```python
from build123d import *

# Parameters (mm, degrees)
SKETCH2_R          = 4.25
CUT_EXTRUDE1_DEPTH = 26.734218465
CHAMFER1_SIZE      = 1
CUT_EXTRUDE2_DEPTH = 26.734218465
CIRPATTERN1_COUNT  = 4


with BuildPart() as part:
    # Sketch1 → Revolve1 (revolve)
    with BuildSketch(Plane.XY, mode=Mode.PRIVATE) as revolve1_sk:
        with BuildLine():
            Line((0, 20.5), (-8, 20.5))
            ThreePointArc((-8, 20.5), (-9.532088886, 19.785575219), (-9.969615506, 18.152703645))
            Line((-9.969615506, 18.152703645), (-8.769638586, 11.347296355))
            ThreePointArc((-8.769638586, 11.347296355), (-9.207165206, 9.714424781), (-10.739254092, 9))
            Line((-10.739254092, 9), (-11, 9))
            Line((-11, 9), (-11, 4))
            Line((-11, 4), (-9.5, 0))
            Line((-9.5, 0), (-8.75, 0))
            Line((-8.75, 0), (0, 8.75))
            Line((0, 8.75), (0, 20.5))
        make_face()
    revolve(revolve1_sk.sketch.rotate(Axis((0, 20.5, 0), (0, -1, 0)), 270), axis=Axis((0, 20.5, 0), (0, -1, 0)))

    # Sketch2 → Cut-Extrude1 (cut, through all)
    with BuildSketch(Plane(origin=(0, 20.5, 0), x_dir=(1, 0, 0), z_dir=(0, 1, 0))):
        with Locations(Location((0, 0, 0), (0, 0, 270))):
            Circle(SKETCH2_R)
    extrude(amount=-CUT_EXTRUDE1_DEPTH, mode=Mode.SUBTRACT)

    # Chamfer1
    chamfer1_edges = [part.edges().sort_by_distance(p)[0] for p in [
        (0, 20.5, -4.25),
    ]]
    chamfer(chamfer1_edges, length=CHAMFER1_SIZE)

    # Sketch3 → Cut-Extrude2 (cut, symmetric)
    with BuildSketch(Plane(origin=(0, 0, 0), x_dir=(0, 0, -1), z_dir=(1, 0, 0))):
        with BuildLine():
            Line((-8.5, 20.5), (-6.974294891, 11.847296355))
            ThreePointArc((-6.974294891, 11.847296355), (-7.411821511, 10.214424781), (-8.943910397, 9.5))
            Line((-8.943910397, 9.5), (-13.5, 9.5))
            Line((-13.5, 9.5), (-13.5, 20.5))
            Line((-13.5, 20.5), (-8.5, 20.5))
        make_face()
    cut_extrude2 = extrude(amount=CUT_EXTRUDE2_DEPTH, both=True, mode=Mode.SUBTRACT)

    # CirPattern1: Cut-Extrude2 ×4 about axis
    cirpattern1_axis = Axis((0, 0, 0), (0, 1, 0))
    for i in range(1, CIRPATTERN1_COUNT):
        add(cut_extrude2.rotate(cirpattern1_axis, i * 360 / CIRPATTERN1_COUNT), mode=Mode.SUBTRACT)


solid = part.part
```
Could you check a few things on this model? Use its own coordinates, in mm. A direction names the side the tool comes from. Round coordinates to 2 decimals unless told otherwise and drop trailing zeros. Loops run counter-clockwise (first coordinate to the right, second up) from the corner with the lowest first, then second, coordinate; pieces in that order, holes last. Notation, with made-up numbers: (15, 17) - (58, 17) arc R14 cw to (58, 29) - close; hole circle Ø4 at (54.5, 48.5). An arc over 180 degrees is marked (long way). Answer in a Markdown table with one row per item. Add a question column.
(1) If we section it at B-B (z = 0): Please give me the cut outline in (x, y), plus the area to 3 significant figures.
(2) I'm going to push flat-ended pins straight in: pin 1 (1.5 mm diameter, centred on y = 13.5, z = 3, fed in from -X); pin 2 (2 mm diameter, centred on x = -2, z = 0, fed in from +Y); pin 3 (1.5 mm diameter, centred on x = -5, y = 17, fed in from +Z); pin 4 (2 mm diameter, centred on x = -3.5, y = 2.5, fed in from +Z). Where does each tip first touch, or does it pass through?
(3) If we section it at C-C (y = 17.25): Please give me the cut outline in (x, z), plus the area to 3 significant figures.
(4) If we section it at D-D (y = 10): Please give me the cut outline in (x, z).
(5) For faces 5 (the face through (7.74, 16.2, -0.08)), 6 (the face through (-0.08, 16.2, -7.74)), 7 (the face through (-6.634, 14.702, -6.604)), 8 (the face through (6.604, 14.702, -6.634)), 9 (the face through (-7.74, 16.2, 0.08)), which set-ups out of +Z, -Z, +X, -X, +Y, -Y let a thin tool reach every point of the face, with its end or its side?
(6) If we section it at A-A (x = 0): Please give me the cut outline in (y, z), plus the area to 3 significant figures.
(7) I need wall thicknesses on line 1 along X through (y, z) = (14, -2.5); line 2 along X through (y, z) = (6.25, 2); line 3 along Z through (x, y) = (-1.75, 16). Which ranges of each line are inside material? Lowest first, please.
(8) If we mould it in two halves opening along Y, with no side actions, what happens to faces 1 (the face through (10.74, 6.46, -2.38)), 2 (the face through (-0.08, 10.23, -7.4)), 3 (the face through (-2.875, 0.194, 9.131)), 4 (the face through (1.7, 20.5, -5.2))? For each: pulls with the +Y half, pulls with the -Y half, needs draft (parallel to the pull), parting line crosses it, or undercut.
Model answer:
| question | item | result |
|---|---|---|
| 1 | outline | (-11, 4) - (-9.5, 0) - (-8.75, 0) - (-4.25, 4.5) - (-4.25, 19.5) - (-5.25, 20.5) - (-8, 20.5) arc R2 ccw to (-8.49, 20.44) - (-6.97, 11.85) arc R2 cw to (-8.94, 9.5) - (-9.42, 9.5) arc R2 cw to (-10.74, 9) - (-11, 9) - close; (4.25, 4.5) - (8.75, 0) - (9.5, 0) - (11, 4) - (11, 9) - (10.74, 9) arc R2 cw to (9.42, 9.5) - (8.94, 9.5) arc R2 cw to (6.97, 11.85) - (8.49, 20.44) arc R2 ccw to (8, 20.5) - (5.25, 20.5) - (4.25, 19.5) - close |
| 1 | area | 175 mm² |
| 2 | pin 1 | stops at x = -7.4 |
| 2 | pin 2 | passes through |
| 2 | pin 3 | stops at z = 8.02 |
| 2 | pin 4 | stops at z = 10.34 |
| 3 | outline | (-7.93, -5.78) arc R9.81 ccw to (-5.78, -7.93) - (5.78, -7.93) arc R9.81 ccw to (7.93, -5.78) - (7.93, 5.78) arc R9.81 ccw to (5.78, 7.93) - (-5.78, 7.93) arc R9.81 ccw to (-7.93, 5.78) - close; hole circle Ø8.5 at (0, 0) |
| 3 | area | 186 mm² |
| 4 | outline | (-7.62, -4.8) arc R9.01 ccw to (-4.8, -7.62) - (4.8, -7.62) arc R9.01 ccw to (7.62, -4.8) - (7.62, 4.8) arc R9.01 ccw to (4.8, 7.62) - (-4.8, 7.62) arc R9.01 ccw to (-7.62, 4.8) - close; hole circle Ø8.5 at (0, 0) |
| 5 | face 5 | +Z, -Z, +X |
| 5 | face 6 | -Z, +X, -X |
| 5 | face 7 | -Z, -X |
| 5 | face 8 | -Z, +X |
| 5 | face 9 | +Z, -Z, -X |
| 6 | outline | (0, -9.5) - (4, -11) - (9, -11) - (9, -10.74) arc R2 cw to (9.5, -9.42) - (9.5, -8.94) arc R2 cw to (11.85, -6.97) - (20.44, -8.49) arc R2 ccw to (20.5, -8) - (20.5, -5.25) - (19.5, -4.25) - (4.5, -4.25) - (0, -8.75) - close; (0, 8.75) - (4.5, 4.25) - (19.5, 4.25) - (20.5, 5.25) - (20.5, 8) arc R2 ccw to (20.44, 8.49) - (11.85, 6.97) arc R2 cw to (9.5, 8.94) - (9.5, 9.42) arc R2 cw to (9, 10.74) - (9, 11) - (4, 11) - (0, 9.5) - close |
| 6 | area | 175 mm² |
| 7 | line 1 | x = -7.35 to -3.44, 3.44 to 7.35 |
| 7 | line 2 | x = -10.82 to -3.75, 3.75 to 10.82 |
| 7 | line 3 | z = -7.71 to -3.87, 3.87 to 7.71 |
| 8 | face 1 | needs draft |
| 8 | face 2 | undercut |
| 8 | face 3 | pulls with the -Y half |
| 8 | face 4 | pulls with the +Y half |
